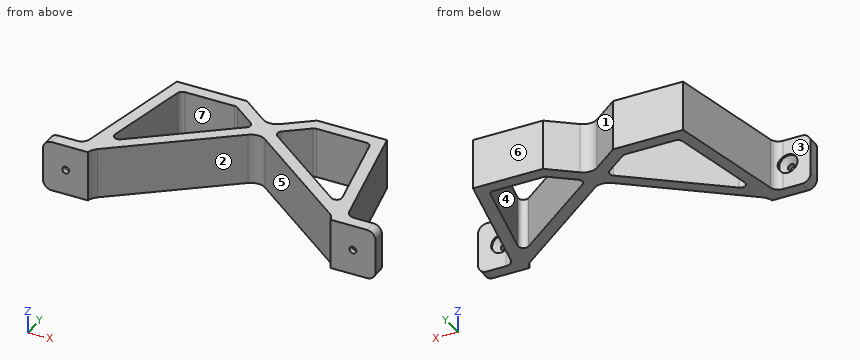
```python
from build123d import *

# Parameters (mm, degrees)
EXTRU_MINCE1_DEPTH      = 14.5
CONG_1_R                = 5
CONG_2_R                = 5
ESQUISSE4_R             = 2
ENL_V_MAT_EXTRU_1_DEPTH = 3
ESQUISSE5_R             = 5.5
ENL_V_MAT_EXTRU_2_DEPTH = 124.143209313
CHANFREIN1_SIZE2        = 3.5
CHANFREIN1_SIZE         = 2.936848709
CONG_3_R                = 8
CONG_4_R                = 3


with BuildPart() as part:
    # Esquisse1 → Extru.-Mince1 (new, symmetric)
    with BuildSketch(Plane.XY):
        Polygon((-95, 0), (-75, 0), (-60, 73), (-20, 73), (75, 0), (70.734848823, -5.550539203), (-22.378866577, 66), (-54.292107606, 66), (-69.292107606, -7), (-95, -7), align=None)
    extrude(amount=EXTRU_MINCE1_DEPTH, both=True)

    # Congé1
    cong_1_edges = [part.edges().sort_by_distance(p)[0] for p in [
        (-95, -3.5, 14.5),
        (-95, -3.5, -14.5),
    ]]
    fillet(cong_1_edges, radius=CONG_1_R)

    # Congé2
    cong_2_edges = [part.edges().sort_by_distance(p)[0] for p in [
        (-75, 0, 0),
    ]]
    fillet(cong_2_edges, radius=CONG_2_R)

    # Esquisse4 → Enlèv. mat.-Extru.1 (cut)
    with BuildSketch(Plane.XZ.offset(7)):
        with Locations((-82, 0)):
            Circle(ESQUISSE4_R)
    extrude(amount=-ENL_V_MAT_EXTRU_1_DEPTH, mode=Mode.SUBTRACT)

    # Esquisse5 → Enlèv. mat.-Extru.2 (cut, through all)
    with BuildSketch(Plane.XZ.offset(4)):
        with Locations((-82, 0)):
            Circle(ESQUISSE5_R)
    extrude(amount=-ENL_V_MAT_EXTRU_2_DEPTH, mode=Mode.SUBTRACT)

    # Chanfrein1
    chanfrein1_edges = [part.edges().sort_by_distance(p)[0] for p in [
        (-87.5, -4, 0),
    ]]
    chanfrein1_side = [part.faces().sort_by_distance(p)[0] for p in [
        (-87.5, -3.941263026, 0),
    ]]
    chamfer(chanfrein1_edges, length=CHANFREIN1_SIZE - 0.0001, length2=CHANFREIN1_SIZE2 - 0.0001, reference=chanfrein1_side[0])  # a hair under: the kernel refuses the full size

    # Symétrie1: part across plane


with BuildPart() as part_1:
    add(part.part)
    add(part.part.mirror(Plane(origin=(0, 0, 0), x_dir=(0, 0, 1), z_dir=(1, 0, 0))))

    # Congé3
    cong_3_edges = [part_1.edges().sort_by_distance(p)[0] for p in [
        (0, 48.803607788, 0),
        (-68.667915266, -3.962263942, 0),
        (0, 57.631578947, 0),
        (68.667915266, -3.962263942, 0),
    ]]
    fillet(cong_3_edges, radius=CONG_3_R)

    # Congé4
    cong_4_edges = [part_1.edges().sort_by_distance(p)[0] for p in [
        (-22.378866577, 66, 0),
        (-54.292107606, 66, 0),
        (5.744227809, 53.217593368, 0),
        (-5.744227809, 53.217593368, 0),
        (66.513829837, 6.520951809, 0),
        (-66.513829837, 6.520951809, 0),
        (54.292107606, 66, 0),
        (22.378866577, 66, 0),
    ]]
    fillet(cong_4_edges, radius=CONG_4_R)


solid = part_1.part
```
Can you work these out from the model? Positions are in its coordinate system, mm. Face numbers are marked on the shaded views. A direction names the side the tool comes from. Coordinates: 2 decimals unless noted, no trailing zeros. Order: outer loops, then holes, each group sorted by start corner. A loop starts at its lowest first (then second) coordinate and runs counter-clockwise, first axis right, second up. Notation, with made-up numbers: (15, 47) - (30, 47) arc R20 cw to (30, 81) - close; hole circle Ø8 at (-30, 32). An arc over 180 degrees is marked (long way). Answer in a Markdown table with one row per item.
1. If I drill on line 1 along Z through (x, y) = (82, -6.2); line 2 along X through (y, z) = (64, -8.5); line 3 along X through (y, z) = (11.5, 0.75), over which ranges is the centre line in solid material (lowest first)?
Reply:
| item | result |
|---|---|
| line 1 | z = -14.5 to -2, 2 to 14.5 |
| line 2 | x = -61.85 to -54.67, -19.78 to -8.29, 8.29 to 19.78, 54.67 to 61.85 |
| line 3 | x = -72.64 to -63.87, -60.03 to -48.55, 48.55 to 60.03, 63.87 to 72.64 |
2. Suppose I cut it at C-C (x = -36). Please give me the cut outline in (y, z), and give its area (3 significant figures).
Reply:
| item | result |
|---|---|
| outline | (21.14, -14.5) - (29.97, -14.5) - (29.97, 14.5) - (21.14, 14.5) - close; (66, -14.5) - (73, -14.5) - (73, 14.5) - (66, 14.5) - close |
| area | 459 mm^2 |
3. Suppose I cut it at B-B (z = 0). Give the number of separate pieces and of enclosed holes in the cut face, and give its area (3 significant figures).
Reply:
| item | result |
|---|---|
| separate pieces | 3 |
| enclosed holes | 2 |
| area | 3,350 mm^2 |
4. For the marked faces 1, 2, 3 and 4, which set-ups out of +Z, -Z, +X, -X, +Y, -Y let a thin tool reach every point of the face, with its end or its side?
Reply:
| item | result |
|---|---|
| face 1 | +Z, -Z, +Y |
| face 2 | +Z, -Z, -Y |
| face 3 | +Z, -Z, -X, +Y |
| face 4 | +Z, -Z |
5. If we mould it in two halves opening along Y, with no side actions, what happens to the marked faces 5, 6 and 7? For each: pulls with the +Y half, pulls with the -Y half, needs draft (parallel to the pull), parting line crosses it, or undercut.
Reply:
| item | result |
|---|---|
| face 5 | pulls with the -Y half |
| face 6 | pulls with the +Y half |
| face 7 | undercut |
6. For pin 1 (1.2 mm diameter, centred on x = -82, z = -0.5, fed in from +Y); pin 2 (1.5 mm diameter, centred on y = 58.5, z = -6, fed in from +X); pin 3 (4 mm diameter, centred on y = 43.5, z = -2, fed in from -X); pin 4 (12 mm diameter, centred on x = 26, z = 6.5, fed in from -Y), each with a flat end and sliding along its axis, tell me the tip position at first contact or that it passes through.
Reply:
| item | result |
|---|---|
| pin 1 | passes through |
| pin 2 | stops at x = 63.13 |
| pin 3 | stops at x = -66.47 |
| pin 4 | stops at y = 24.21 |
